Can you work these out from the model? Positions are in its coordinate system, mm. A direction names the side the tool comes from. Give positions to 0.01 mm unless a question says otherwise; leave off trailing zeros. Loops run counter-clockwise (first coordinate to the right, second up) from the corner with the lowest first, then second, coordinate; pieces in that order, holes last. Notation, with made-up numbers: (16.5, 29.5) -> (71.5, 29.5) arc R31 cw to (71.5, 64.5) -> close; hole circle Ø6 at (-34.75, -12.5). An arc over 180 degrees is marked (long way). Return JSON: item names as keys, results as strings. Group by question number.
Q1. Suppose I cut it at B-B, the plane y = 101.5. Please give me the cut outline in (x, z).
Q2. Suppose I cut it at C-C, the plane x = -33.5. Please give me the cut outline in (y, z).
Q3. Suppose I cut it at A-A, the plane x = 66. Count the separate pieces of the cut face and the enclosed holes in it, and give its area (3 significant figures).
Q4. Suppose I cut it at D-D, the plane y = 51.5. Please give me the cut outline in (x, z).
Q5. Which directions (+Z, -Z, +X, -X, +Y, -Y) give clear straight access to the entire face, cutting with the end or side of a thin tool? Please do faces 1 (the flat face through (48.275, 86, 0)), 2 (the flat face through (4, 68, -0.801)), 3 (the flat face through (55, 82.65, -2)).
Q6. I need wall thicknesses on line 1 along X through (y, z) = (66, -0.35); line 2 along Y through (x, z) = (66, 0.05). Which ranges of each line are inside material? Lowest first, please. Write a range as [from, to].
Q7. Will these pins go through, and if not, where does the flat tip stop? pin 1 (4 mm diameter, centred on x = 66, y = 4, fed in from -Z); pin 2 (0.7 mm diameter, centred on y = 63, z = 2, fed in from +X); pin 3 (1.6 mm diameter, centred on y = 67.5, z = 2, fed in from -X).
Q8. Thinking about a two-plate mould opening in X: for faces 4 (the cylindrical face through (64.57, 3.55, -0.01)), 5 (the flat face through (62.5, 17, 2)), 6 (the flat face through (49, 71.8, -3)), which applies, pulls with the +X half, pulls with the -X half, needs draft (parallel to the pull), parting line crosses it, or undercut?
```python
from build123d import *
from build123d.topology import SkipClean

# Parameters (mm, degrees)
SKETCH1_W                     = 70
SKETCH1_H                     = 70
GREEN_PCB_DEPTH               = 0.8
SKETCH2_R                     = 1.5
MOUNTING_HOLES_DEPTH          = 100.007878474
SCREW_GROUNDS_DEPTH           = 0.801
SCREW_GROUNDS_DEPTH_BACK      = 0.801
SKETCH3_R                     = 3.6
SKETCH3_R_2                   = 1.5
SKETCH4_W                     = 9.5
SKETCH4_H                     = 7.9
ANTENNA1_DEPTH                = 1.8
SKETCH10_W                    = 1.25
SKETCH10_H                    = 4.5
ANTENNA2_DEPTH                = 2
SKETCH5_R                     = 2.7
ANTENNA3_DEPTH                = 2.6
SKETCH6_R                     = 3.85
ANTENNA4_DEPTH                = 2.25
ANTENNA5_DEPTH                = 6
SKETCH8_R                     = 3.15
ANTENNA6_DEPTH                = 2.4
SKETCH9_W                     = 6.45
SKETCH9_H                     = 6.45
ANTENNA7_DEPTH                = 1.45
SKETCH11_W                    = 40
SKETCH11_H                    = 0.8
ANTENNA_PCB_DEPTH             = 31
SKETCH19_W                    = 1
SKETCH19_H                    = 4
ANTENNA8_DEPTH                = 1.675
SKETCH12_W                    = 55
SKETCH12_H                    = 28
LCD_DEPTH                     = 2.5
SKETCH13_W                    = 11.25
SKETCH13_H                    = 6
OPTION_SWITCH_DEPTH           = 2.25
SKETCH14_W                    = 7.8
SKETCH14_H                    = 7.5
USB_PORT_DEPTH                = 2.6
USB_BODY_DEPTH                = 3.5
USB_TENSION_RELIEF_DEPTH      = 6
USB_TENSION_RELIEF_DEPTH_BACK = 6
SKETCH17_R                    = 3.5
SKETCH18_R                    = 2
USB_CORD_DEPTH                = 15


with BuildPart() as part:
    # Sketch1 → Green PCB (new, symmetric)
    with BuildSketch(Plane.XY):
        with Locations((35, 35)):
            Rectangle(SKETCH1_W, SKETCH1_H)
    extrude(amount=GREEN_PCB_DEPTH, both=True)

    # Sketch2 → Mounting Holes (cut, through all)
    with BuildSketch(Plane.XY.offset(0.8)):
        with Locations((4, 4)):
            Circle(SKETCH2_R)
        with Locations((66, 4)):
            Circle(SKETCH2_R)
        with Locations((66, 66)):
            Circle(SKETCH2_R)
        with Locations((4, 66)):
            Circle(SKETCH2_R)
    extrude(amount=-MOUNTING_HOLES_DEPTH, mode=Mode.SUBTRACT)

    # Sketch3 → Screw Grounds (add, two sides: drawn at the far end of the back side and taken through both)
    # profile 1 of 4: a face of its own
    with BuildSketch(Plane.XY.offset(-SCREW_GROUNDS_DEPTH_BACK)):
        with Locations(Location((4, 66, 0), (0, 0, 180))):
            Circle(SKETCH3_R)
        with Locations(Location((4, 66, 0), (0, 0, 180))):
            Circle(SKETCH3_R_2, mode=Mode.SUBTRACT)
    # profile 2 of 4: a face of its own
    with BuildSketch(Plane.XY.offset(-SCREW_GROUNDS_DEPTH_BACK)):
        with Locations(Location((66, 66, 0), (0, 0, 180))):
            Circle(SKETCH3_R)
        with Locations(Location((66, 66, 0), (0, 0, 180))):
            Circle(SKETCH3_R_2, mode=Mode.SUBTRACT)
    # profile 3 of 4: a face of its own
    with BuildSketch(Plane.XY.offset(-SCREW_GROUNDS_DEPTH_BACK)):
        with Locations(Location((66, 4, 0), (0, 0, 180))):
            Circle(SKETCH3_R)
        with Locations(Location((66, 4, 0), (0, 0, 180))):
            Circle(SKETCH3_R_2, mode=Mode.SUBTRACT)
    # profile 4 of 4: a face of its own
    with BuildSketch(Plane.XY.offset(-SCREW_GROUNDS_DEPTH_BACK)):
        with Locations(Location((4, 4, 0), (0, 0, 180))):
            Circle(SKETCH3_R)
        with Locations(Location((4, 4, 0), (0, 0, 180))):
            Circle(SKETCH3_R_2, mode=Mode.SUBTRACT)
    extrude(amount=SCREW_GROUNDS_DEPTH + SCREW_GROUNDS_DEPTH_BACK)

    # Sketch4 → Antenna1 (add)
    with BuildSketch(Plane(origin=(0, 70, 0), x_dir=(1, 0, 0), z_dir=(0, 1, 0))):
        with Locations((51.5, 1.15)):
            Rectangle(SKETCH4_W, SKETCH4_H)
    extrude(amount=ANTENNA1_DEPTH)

    # Sketch10 → Antenna2 (add)
    with BuildSketch(Plane.XY.offset(2.8)):
        with Locations((47.375, 67.75)):
            Rectangle(SKETCH10_W, SKETCH10_H)
        with Locations((55.625, 67.75)):
            Rectangle(SKETCH10_W, SKETCH10_H)
    extrude(amount=-ANTENNA2_DEPTH)

    # Sketch5 → Antenna3 (add)
    with BuildSketch(Plane(origin=(0, 71.8, 0), x_dir=(1, 0, 0), z_dir=(0, 1, 0))):
        with Locations(Location((51.5, 1.15, 0), (0, 0, 270))):
            Circle(SKETCH5_R)
    extrude(amount=ANTENNA3_DEPTH)

    # Sketch6 → Antenna4 (add)
    with SkipClean():  # the faces are left unmerged after this step: merging them gives an invalid solid
        with BuildSketch(Plane(origin=(0, 74.4, 0), x_dir=(1, 0, 0), z_dir=(0, 1, 0))):
            with Locations(Location((51.5, 1.15, 0), (0, 0, 270))):
                Circle(SKETCH6_R)
        extrude(amount=ANTENNA4_DEPTH)

    # Sketch7 → Antenna5 (add)
    with SkipClean():  # the faces are left unmerged after this step: merging them gives an invalid solid
        with BuildSketch(Plane(origin=(0, 76.65, 0), x_dir=(1, 0, 0), z_dir=(0, 1, 0))):
            Polygon((49.219466437, -2.8), (53.780533563, -2.8), (56.061067127, 1.15), (53.780533563, 5.1), (49.219466437, 5.1), (46.938932873, 1.15), align=None)
        extrude(amount=ANTENNA5_DEPTH)

    # Sketch8 → Antenna6 (add)
    with SkipClean():  # the faces are left unmerged after this step: merging them gives an invalid solid
        with BuildSketch(Plane(origin=(0, 82.65, 0), x_dir=(1, 0, 0), z_dir=(0, 1, 0))):
            with Locations(Location((51.5, 1.15, 0), (0, 0, 270))):
                Circle(SKETCH8_R)
        extrude(amount=ANTENNA6_DEPTH)

    # Sketch9 → Antenna7 (add)
    with SkipClean():  # the faces are left unmerged after this step: merging them gives an invalid solid
        with BuildSketch(Plane(origin=(0, 85.05, 0), x_dir=(1, 0, 0), z_dir=(0, 1, 0))):
            with Locations((51.5, 1.15)):
                Rectangle(SKETCH9_W, SKETCH9_H)
        extrude(amount=ANTENNA7_DEPTH)

    # Sketch11 → Antenna PCB (add)
    with SkipClean():  # the faces are left unmerged after this step: merging them gives an invalid solid
        with BuildSketch(Plane(origin=(0, 86.5, 0), x_dir=(1, 0, 0), z_dir=(0, 1, 0))):
            with Locations((51.5, 0)):
                Rectangle(SKETCH11_W, SKETCH11_H)
        extrude(amount=ANTENNA_PCB_DEPTH)

    # Sketch19 → Antenna8 (add)
    with SkipClean():  # the faces are left unmerged after this step: merging them gives an invalid solid
        with BuildSketch(Plane.XY.offset(2.075)):
            with Locations((48.775, 88.5)):
                Rectangle(SKETCH19_W, SKETCH19_H)
            with Locations((54.225, 88.5)):
                Rectangle(SKETCH19_W, SKETCH19_H)
        extrude(amount=-ANTENNA8_DEPTH)

    # Sketch12 → LCD (add)
    with SkipClean():  # the faces are left unmerged after this step: merging them gives an invalid solid
        with BuildSketch(Plane.XY.offset(0.8)):
            with Locations((35, 17.5)):
                Rectangle(SKETCH12_W, SKETCH12_H)
        extrude(amount=LCD_DEPTH)

    # Sketch13 → Option Switch (add)
    with SkipClean():  # the faces are left unmerged after this step: merging them gives an invalid solid
        with BuildSketch(Plane.XY.offset(0.8)):
            with Locations((26.875, 63.5)):
                Rectangle(SKETCH13_W, SKETCH13_H)
        extrude(amount=OPTION_SWITCH_DEPTH)

    # Sketch14 → USB Port (add)
    with SkipClean():  # the faces are left unmerged after this step: merging them gives an invalid solid
        with BuildSketch(Plane(origin=(0, 0, -0.8), x_dir=(-1, 0, 0), z_dir=(0, 0, -1))):
            with Locations((-0.1, 12.75)):
                Rectangle(SKETCH14_W, SKETCH14_H)
        extrude(amount=USB_PORT_DEPTH)

    # Sketch16 → USB Body (add, symmetric)
    with BuildSketch(Plane(origin=(0, 0, -2.1), x_dir=(-1, 0, 0), z_dir=(0, 0, -1))):
        with BuildLine():
            Line((19.3, 7.25), (3.8, 7.25))
            Line((3.8, 7.25), (3.8, 18.25))
            Line((3.8, 18.25), (19.3, 18.25))
            ThreePointArc((19.3, 18.25), (24.8, 12.75), (19.3, 7.25))
        make_face()
    extrude(amount=USB_BODY_DEPTH, both=True)

    # Sketch17 → USB Tension Relief (add, two sides: drawn at the far end of the back side and taken through both)
    with BuildSketch(Plane.ZY.offset(24.8).offset(-USB_TENSION_RELIEF_DEPTH_BACK)):
        with Locations((-2.1, 12.75)):
            Circle(SKETCH17_R)
    extrude(amount=USB_TENSION_RELIEF_DEPTH + USB_TENSION_RELIEF_DEPTH_BACK)

    # Sketch18 → USB Cord (add)
    with BuildSketch(Plane.ZY.offset(30.8)):
        with Locations((-2.1, 12.75)):
            Circle(SKETCH18_R)
    extrude(amount=USB_CORD_DEPTH)


solid = part.part
```
Ans:
{
 "1": {"outline": "(31.5, -0.4) -> (71.5, -0.4) -> (71.5, 0.4) -> (31.5, 0.4) -> close"},
 "2": {"outline": "circle Ø4 at (12.75, -2.1)"},
 "3": {"separate pieces": "4", "enclosed holes": "0", "area": "127 mm^2"},
 "4": {"outline": "(0, -0.8) -> (70, -0.8) -> (70, 0.8) -> (0, 0.8) -> close"},
 "5": {"face 1": "+Z, -X", "face 2": "-Z, +X, -X, +Y", "face 3": "none"},
 "6": {"line 1": "x = [0, 2.5], [5.5, 64.5], [67.5, 70]", "line 2": "y = [0, 2.5], [5.5, 64.5], [67.5, 70], [86.5, 117.5]"},
 "7": {"pin 1": "stops at z = -0.8", "pin 2": "stops at x = 32.5", "pin 3": "stops at x = 46.75"},
 "8": {"face 4": "undercut", "face 5": "pulls with the +X half", "face 6": "needs draft"}
}
